```python
from build123d import *

# Parameters (mm, degrees)
BOSS_EXTRUDE1_DEPTH = 9
BOSS_EXTRUDE2_DEPTH = 12
BOSS_EXTRUDE3_DEPTH = 19
BOSS_EXTRUDE4_DEPTH = 37
CUT_EXTRUDE1_DEPTH  = 6


with BuildPart() as part:
    # Sketch1 → Boss-Extrude1 (new body)
    with BuildSketch(Plane(origin=(0, 0, 0), x_dir=(1, 0, 0), z_dir=(0, 1, 0))):
        with BuildLine():
            Line((1.1176, 2.780970186), (1.1176, 8.7884))
            Line((1.1176, 8.7884), (-9.0424, 8.7884))
            Line((-9.0424, 8.7884), (-9.0424, 1.1684))
            ThreePointArc((-9.0424, 1.1684), (-8.736471312, -10.147543841), (1.1176, -15.719029814))
            Line((1.1176, -15.719029814), (1.1176, -11.219029814))
            ThreePointArc((1.1176, -11.219029814), (-5.8824, -4.219029814), (1.1176, 2.780970186))
        make_face()
        with BuildLine():
            Line((11.2776, 8.7884), (1.1176, 8.7884))
            Line((1.1176, 8.7884), (1.1176, 2.780970186))
            ThreePointArc((1.1176, 2.780970186), (6.067347468, 0.730717654), (8.1176, -4.219029814))
            ThreePointArc((8.1176, -4.219029814), (6.067347468, -9.168777282), (1.1176, -11.219029814))
            Line((1.1176, -11.219029814), (1.1176, -15.719029814))
            ThreePointArc((1.1176, -15.719029814), (10.971671312, -10.147543841), (11.2776, 1.1684))
            Line((11.2776, 1.1684), (11.2776, 8.7884))
        make_face()
    extrude(amount=BOSS_EXTRUDE1_DEPTH)

    # Sketch1_3 → Boss-Extrude2 (add)
    with BuildSketch(Plane(origin=(0, 0, 0), x_dir=(1, 0, 0), z_dir=(0, 1, 0))):
        with BuildLine():
            ThreePointArc((8.1176, -4.219029814), (6.067347468, 0.730717654), (1.1176, 2.780970186))
            Line((1.1176, 2.780970186), (1.1176, -0.409029814))
            ThreePointArc((1.1176, -0.409029814), (3.811676836, -1.524952978), (4.9276, -4.219029814))
            ThreePointArc((4.9276, -4.219029814), (3.811676836, -6.91310665), (1.1176, -8.029029814))
            Line((1.1176, -8.029029814), (1.1176, -11.219029814))
            ThreePointArc((1.1176, -11.219029814), (6.067347468, -9.168777282), (8.1176, -4.219029814))
        make_face()
        with BuildLine():
            Line((1.1176, -0.409029814), (1.1176, 2.780970186))
            ThreePointArc((1.1176, 2.780970186), (-5.8824, -4.219029814), (1.1176, -11.219029814))
            Line((1.1176, -11.219029814), (1.1176, -8.029029814))
            ThreePointArc((1.1176, -8.029029814), (-2.6924, -4.219029814), (1.1176, -0.409029814))
        make_face()
    extrude(amount=BOSS_EXTRUDE2_DEPTH)

    # Sketch1_4 → Boss-Extrude3 (add)
    with BuildSketch(Plane(origin=(0, 0, 0), x_dir=(1, 0, 0), z_dir=(0, 1, 0))):
        with BuildLine():
            ThreePointArc((4.9276, -4.219029814), (3.811676836, -1.524952978), (1.1176, -0.409029814))
            Line((1.1176, -0.409029814), (1.1176, -1.219029814))
            ThreePointArc((1.1176, -1.219029814), (3.238920344, -2.09770947), (4.1176, -4.219029814))
            ThreePointArc((4.1176, -4.219029814), (3.238920344, -6.340350157), (1.1176, -7.219029814))
            Line((1.1176, -7.219029814), (1.1176, -8.029029814))
            ThreePointArc((1.1176, -8.029029814), (3.811676836, -6.91310665), (4.9276, -4.219029814))
        make_face()
        with BuildLine():
            Line((1.1176, -1.219029814), (1.1176, -0.409029814))
            ThreePointArc((1.1176, -0.409029814), (-2.6924, -4.219029814), (1.1176, -8.029029814))
            Line((1.1176, -8.029029814), (1.1176, -7.219029814))
            ThreePointArc((1.1176, -7.219029814), (-1.8824, -4.219029814), (1.1176, -1.219029814))
        make_face()
    extrude(amount=BOSS_EXTRUDE3_DEPTH)

    # Sketch1_5 → Boss-Extrude4 (add)
    with BuildSketch(Plane(origin=(0, 0, 0), x_dir=(1, 0, 0), z_dir=(0, 1, 0))):
        with BuildLine():
            ThreePointArc((4.1176, -4.219029814), (3.238920344, -2.09770947), (1.1176, -1.219029814))
            Line((1.1176, -1.219029814), (1.1176, -7.219029814))
            ThreePointArc((1.1176, -7.219029814), (3.238920344, -6.340350157), (4.1176, -4.219029814))
        make_face()
        with BuildLine():
            Line((1.1176, -7.219029814), (1.1176, -1.219029814))
            ThreePointArc((1.1176, -1.219029814), (-1.8824, -4.219029814), (1.1176, -7.219029814))
        make_face()
    extrude(amount=BOSS_EXTRUDE4_DEPTH)

    # Sketch2 → Cut-Extrude1 (cut)
    with BuildSketch(Plane(origin=(0, 0, 0), x_dir=(-1, 0, 0), z_dir=(0, -1, 0))):
        with BuildLine():
            Line((9.0424, 1.1684), (9.0424, 8.7884))
            Line((9.0424, 8.7884), (-11.2776, 8.7884))
            Line((-11.2776, 8.7884), (-11.2776, 1.1684))
            ThreePointArc((-11.2776, 1.1684), (-1.1176, 7.280970186), (9.0424, 1.1684))
        make_face()
    extrude(amount=-CUT_EXTRUDE1_DEPTH, mode=Mode.SUBTRACT)


solid = part.part
```
Check sheet for the modelled part. Datum: model origin and axes. Units: mm. A direction names the side the tool comes from. Round coordinates to 2 decimals unless told otherwise and drop trailing zeros. Loops run counter-clockwise (first coordinate to the right, second up) from the corner with the lowest first, then second, coordinate; pieces in that order, holes last. Notation, with made-up numbers: (72.25, -15.75) - (115.25, -15.75) arc R35 cw to (115.25, 19.25) - close; hole circle Ø9 at (-9.5, -36). An arc over 180 degrees is marked (long way). Answer as a JSON object with one key per item and string values. Group by question number.
Q1. Set-up check for faces 1 (the face through (-9.042, 7, -5)), 2 (the face through (1, 7, -8.788)), 3 (the face through (6, 9, -2)), 4 (the face through (11.278, 7, -5)), 5 (the face through (1, 6, -8)): record each of +Z, -Z, +X, -X, +Y, -Y from which the full face is reachable in a straight line by a thin tool's end or side.
Q2. Sectioned sample at B-B, the plane x = -4. Enter the section's corners in (y, z).
Q3. Sectioned sample at A-A, the plane z = -4.5. Enter the section's corners in (x, y), plus the area to 3 significant figures.
Q4. Sectioned sample at C-C, the plane y = 29. Enter the section's corners in (x, z).
Q5. Sectioned sample at D-D, the plane z = 10. Enter the section's corners in (x, y), plus the area to 3 significant figures.
Q6. Scan lines: line 1 along Y through (x, z) = (4.5, 13.5); line 2 along Y through (x, z) = (4, -0.5); line 3 along Z through (x, y) = (3, 30.5). Record each from-to range of solid material in increasing order. Write a range as [from, to].
Q7. Gauge pin test, flat ends, axial feed: P1, Ø2, axis at x = 7.5, z = -3.5, coming from the +Y side; P2, Ø10, axis at y = 23.5, z = 8, coming from the -X side; P3, Ø1.5, axis at y = 7.5, z = -4, coming from the +X side. Record the tip position at first contact, or that the pin passes through.
Solution:
{
 "1": {"face 1": "-Z, -X, +Y, -Y", "face 2": "-Z, +X, -X, +Y, -Y", "face 3": "+Y", "face 4": "-Z, +X, +Y, -Y", "face 5": "-Z, -Y"},
 "2": {"outline": "(0, -6.08) - (6, -6.08) - (6, -8.79) - (9, -8.79) - (9, -0.56) - (12, -0.56) - (12, 9) - (9, 9) - (9, 14.52) - (0, 14.52) - close"},
 "3": {"outline": "(-9.04, 6) - (-6.38, 6) - (-6.38, 0) - (8.62, 0) - (8.62, 6) - (11.28, 6) - (11.28, 9) - (-9.04, 9) - close", "area": "151 mm²"},
 "4": {"outline": "circle Ø6 at (1.12, 4.22)"},
 "5": {"outline": "(-8.82, 0) - (11.06, 0) - (11.06, 9) - (5.06, 9) - (5.06, 12) - (-2.83, 12) - (-2.83, 9) - (-8.82, 9) - close", "area": "203 mm²"},
 "6": {"line 1": "y = [0, 9]", "line 2": "y = [0, 12]", "line 3": "z = [1.88, 6.55]"},
 "7": {"P1": "stops at y = 9", "P2": "stops at x = -2.34", "P3": "stops at x = 11.28"}
}
